Geometry: see drawing. Coordinates: mm, zero at the bounding-box minimum. Give positions to 0.01 mm unless a question says otherwise; leave off trailing zeros. Loops run counter-clockwise (first coordinate to the right, second up) from the corner with the lowest first, then second, coordinate; pieces in that order, holes last. Notation, with made-up numbers: (-12, -9.75) -> (8, -9.75) arc R34 ccw to (8, 29.25) -> close; hole circle Ø9 at (44, 33.5). An arc over 180 degrees is marked (long way). Answer in a Markdown table with one row per item. Add a question column.
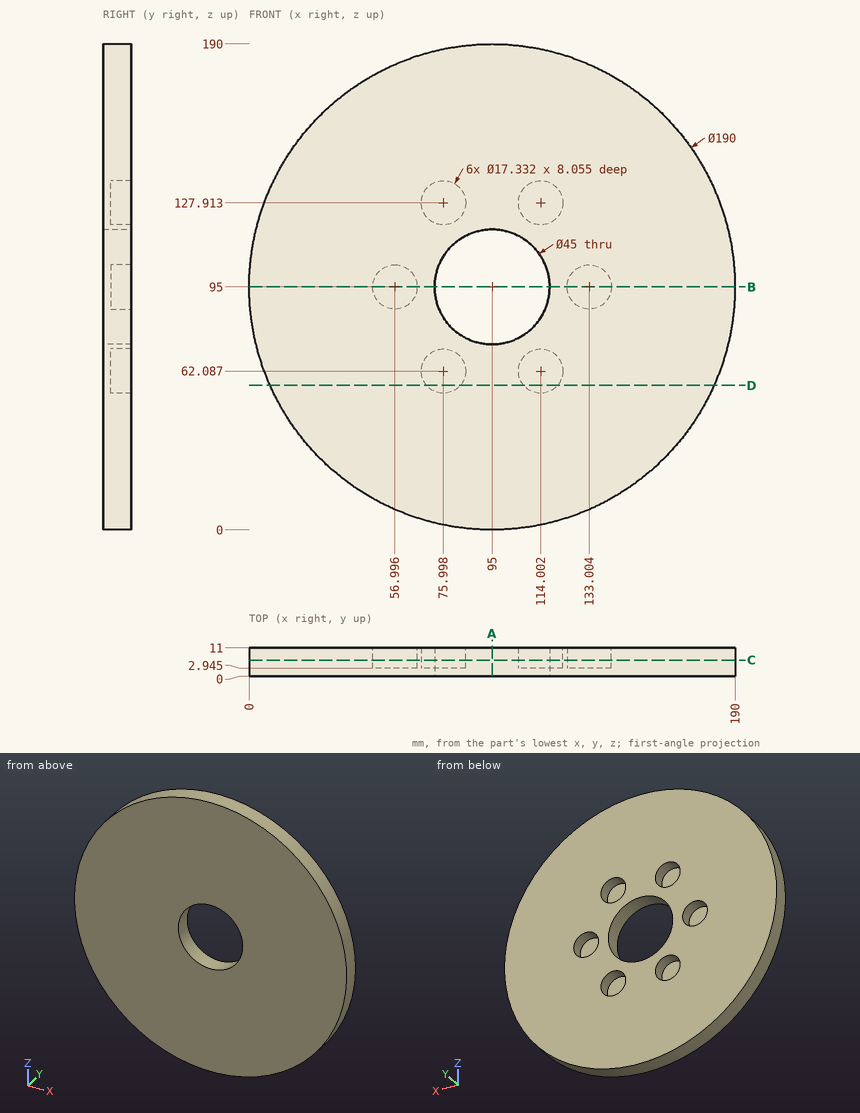
1) Material intervals for line 1 along X through (y, z) = (7.5, 95); line 2 along X through (y, z) = (3, 127) (1 decimal); line 3 along Z through (x, y) = (118, 8.5) (1 decimal), sorted ascending.
2) Section B-B on z = 95. Output: boundary loops of the cut face in (x, y) (1 decimal), and give its area (3 significant figures).
3) Pin query (flat end, axial travel): pin 1 (14 mm diameter, centred on x = 115, z = 127.5, fed in from +Y) (1 decimal); pin 2 (2 mm diameter, centred on y = 7.5, z = 112.5, fed in from +X); pin 3 (1 mm diameter, centred on y = 4.5, z = 170.5, fed in from +X). Return the tip coordinate at first contact, or that it passes through.
4) Section A-A on x = 95. Output: boundary loops of the cut face in (y, z).
5) Section C-C on y = 6.25. Output: boundary loops of the cut face in (x, z) (1 decimal).
6) Section D-D on z = 56.5. Output: boundary loops of the cut face in (x, y) (1 decimal), and give its area (3 significant figures).
Working result:
| question | item | result |
|---|---|---|
| 1 | line 1 | x = 0 to 48.33, 65.66 to 72.5, 117.5 to 124.34, 141.67 to 190 |
| 1 | line 2 | x = 5.6 to 67.4, 84.6 to 105.4, 122.6 to 184.4 |
| 1 | line 3 | z = 2.8 to 54.4, 69.8 to 120.2, 135.6 to 187.2 |
| 2 | outline | (0, 0) -> (72.5, 0) -> (72.5, 11) -> (65.7, 11) -> (65.7, 2.9) -> (48.3, 2.9) -> (48.3, 11) -> (0, 11) -> close; (117.5, 0) -> (190, 0) -> (190, 11) -> (141.7, 11) -> (141.7, 2.9) -> (124.3, 2.9) -> (124.3, 11) -> (117.5, 11) -> close |
| 2 | area | 1,320 mm2 |
| 3 | pin 1 | stops at y = 2.9 |
| 3 | pin 2 | stops at x = 188.56 |
| 3 | pin 3 | stops at x = 153.31 |
| 4 | outline | (0, 0) -> (11, 0) -> (11, 72.5) -> (0, 72.5) -> close; (0, 117.5) -> (11, 117.5) -> (11, 190) -> (0, 190) -> close |
| 5 | outline | circle Ø190 at (95, 95); hole circle Ø17.3 at (57, 95); hole circle Ø17.3 at (76, 62.1); hole circle Ø17.3 at (76, 127.9); hole circle Ø45 at (95, 95); hole circle Ø17.3 at (114, 62.1); hole circle Ø17.3 at (114, 127.9); hole circle Ø17.3 at (133, 95) |
| 6 | outline | (8.2, 0) -> (181.8, 0) -> (181.8, 11) -> (120.6, 11) -> (120.6, 2.9) -> (107.4, 2.9) -> (107.4, 11) -> (82.6, 11) -> (82.6, 2.9) -> (69.4, 2.9) -> (69.4, 11) -> (8.2, 11) -> close |
| 6 | area | 1,700 mm2 |
